Verification items for the finished model (mm, model axes). Coordinates: 2 decimals unless noted, no trailing zeros. Write each loop counter-clockwise with the first axis right and the second up, starting at its lowest first coordinate (ties: lowest second). Pieces come first, ordered by that corner, then holes. Notation, with made-up numbers: (69, 71) -> (89, 71) arc R25 ccw to (89, 92) -> close; hole circle Ø4 at (1, -7.75). An arc over 180 degrees is marked (long way). Answer in a Markdown table with one row per item.
```python
from build123d import *

# Parameters (mm, degrees)
F1_DEPTH = 38.1
F2_R     = 2.54
F3_R     = 2.54


with BuildPart() as f1:
    # F0 (on Front) → F1 (new body, symmetric)
    with BuildSketch(Plane.XZ):
        Polygon((21.662317, 50.8), (-50.8, 50.8), (-50.8, -50.8), (50.8, -50.8), (50.8, 9.187076), align=None)
    extrude(amount=F1_DEPTH, both=True)

    # F2
    f2_edges = [f1.edges().sort_by_distance(p)[0] for p in [
        (-50.8, -38.1, 0),
        (-14.568841, -38.1, 50.8),
    ]]
    fillet(f2_edges, radius=F2_R)

    # F3
    f3_edges = [f1.edges().sort_by_distance(p)[0] for p in [
        (50.8, -38.1, -20.806462),
    ]]
    fillet(f3_edges, radius=F3_R)


solid = f1.part
```
1. Section check C-C, the plane x = 36. Record the boundary of the cut face in (y, z).
Geometry says:
| item | result |
|---|---|
| outline | (-38.1, -50.8) -> (38.1, -50.8) -> (38.1, 30.32) -> (-38.1, 30.32) -> close |
2. Thickness scan on line 1 (X direction, y = 17.5, z = 31); line 2 (Z direction, x = 35, y = -5); line 3 (X direction, y = 29.5, z = 39). Record the ranges inside material, lowest first. Write a range as from..to.
Geometry says:
| item | result |
|---|---|
| line 1 | -50.8..35.53 |
| line 2 | -50.8..31.75 |
| line 3 | -50.8..29.92 |
3. Section check A-A, the plane y = 19. Record the boundary of the cut face in (x, z).
Geometry says:
| item | result |
|---|---|
| outline | (-50.8, -50.8) -> (50.8, -50.8) -> (50.8, 9.19) -> (21.66, 50.8) -> (-50.8, 50.8) -> close |
4. Section check B-B, the plane z = 32.5. Record the boundary of the cut face in (x, y), plus the area to 3 significant figures.
Geometry says:
| item | result |
|---|---|
| outline | (-50.8, -35.56) arc R2.54 ccw to (-48.26, -38.1) -> (34.48, -38.1) -> (34.48, 38.1) -> (-50.8, 38.1) -> close |
| area | 6,500 mm^2 |
5. Depth check by flat-ended pin: P1, Ø12, axis at y = 8, z = 25, coming from the +X side; P2, Ø6, axis at x = 35.5, y = 15.5, coming from the +Z side. Enter the tip coordinate at first touch or a pass-through.
Geometry says:
| item | result |
|---|---|
| P1 | x = 43.93 |
| P2 | z = 35.32 |
